Drawing for the job (mm, zero at the part's lowest x, y, z). Round coordinates to 2 decimals unless told otherwise and drop trailing zeros. Order: outer loops, then holes, each group sorted by start corner. A loop starts at its lowest first (then second) coordinate and runs counter-clockwise, first axis right, second up. Notation, with made-up numbers: (34.5, 46.25) - (87.5, 46.25) arc R10 ccw to (87.5, 60.25) - close; hole circle Ø3 at (9, -7.5). An arc over 180 degrees is marked (long way). Answer as a JSON object with one key per item and string values.
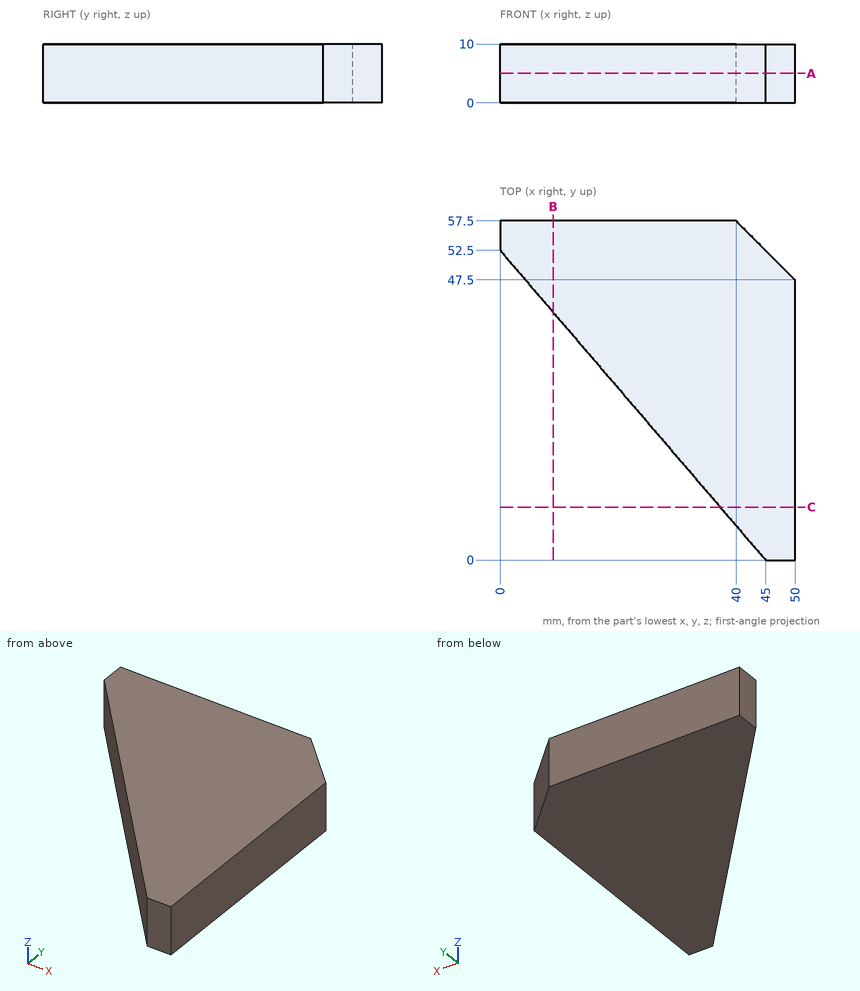
Item 1: Drop flat-ended pins along their axis: P1, Ø2, axis at x = 16, z = 4, coming from the -Y side; P2, Ø1, axis at x = 43.5, z = 6.5, coming from the +Y side; P3, Ø2, axis at x = 43, z = 7.5, coming from the -Y side. Give the stop position or say it passes through.
Taken from the geometry:
{"P1": "y = 32.67", "P2": "y = 54.5", "P3": "y = 1.17"}
Item 2: Cut at A-A (z = 5). Write the cut outline in (x, y), plus the area to 3 significant figures.
Taken from the geometry:
{"outline": "(0, 52.5) - (45, 0) - (50, 0) - (50, 47.5) - (40, 57.5) - (0, 57.5) - close", "area": "1,640 mm2"}
Item 3: Cut at C-C (y = 9). Write the cut outline in (x, z).
Taken from the geometry:
{"outline": "(37.29, 0) - (50, 0) - (50, 10) - (37.29, 10) - close"}
Item 4: Probe L1, parallel to X at y = 52.5, z = 7; L2, parallel to X at y = 32.5, z = 9; L3, parallel to Y at x = 3, z = 0.5. List the from-to ranges inside material, lowest first. Write a range as from..to.
Taken from the geometry:
{"L1": "0..45", "L2": "17.14..50", "L3": "49..57.5"}
Item 5: Cut at B-B (x = 9). Write the cut outline in (y, z), plus the area to 3 significant figures.
Taken from the geometry:
{"outline": "(42, 0) - (57.5, 0) - (57.5, 10) - (42, 10) - close", "area": "155 mm2"}
